from build123d import *

# Parameters (mm, degrees)
SKETCH1_R                       = 24.13
SKETCH1_R_2                     = 2.5
BOSS_EXTRUDE1_DEPTH             = 6.35
F_5_32_0_15625_DIAMETER_HOLE1_D = 3.96875


with BuildPart() as part:
    # Sketch1 → Boss-Extrude1 (new body)
    with BuildSketch(Plane(origin=(0, 0, 0), x_dir=(1, 0, 0), z_dir=(0, 1, 0))):
        Circle(SKETCH1_R)
        with Locations((19.2, 0)):
            Circle(SKETCH1_R_2, mode=Mode.SUBTRACT)
        with Locations((-9.6, 16.627687753)):
            Circle(SKETCH1_R_2, mode=Mode.SUBTRACT)
        with Locations((-9.6, -16.627687753)):
            Circle(SKETCH1_R_2, mode=Mode.SUBTRACT)
    extrude(amount=BOSS_EXTRUDE1_DEPTH)

    # 5/32 (0.15625) Diameter Hole1 (through all)
    with Locations(Plane(origin=(0, 6.35, 0), x_dir=(1, 0, 0), z_dir=(0, 1, 0))):
        with Locations((4.7625, 8.248891971), (-4.7625, 8.248891971), (-9.525, 0), (-4.7625, -8.248891971), (4.7625, -8.248891971), (9.525, 0)):
            Hole(F_5_32_0_15625_DIAMETER_HOLE1_D / 2)


solid = part.part
Build history of the part. All positions in model axes, mm. Give positions to 0.01 mm unless a question says otherwise; leave off trailing zeros. Order: outer loops, then holes, each group sorted by start corner. A loop starts at its lowest first (then second) coordinate and runs counter-clockwise, first axis right, second up. Notation, with made-up numbers: M 32.25,-14.75 L 44.25,-14.75 A19 ccw 44.25,4.25 Z; hole C 25.5,83 d3. An arc over 180 degrees is marked long. Use one line per item in the form item = value.
Q1. Pull direction X, two halves, no side cores. Call faces 1 (the cylindrical face through (5.021, 3.131, -10.216)), 2 (the cylindrical face through (23.016, 3.131, -7.248)), 3 (the flat face through (0, 6.35, 0)), 4 (the cylindrical face through (-7.543, 3.131, -0.087)): released by +X, released by -X, zero draft, split by the parting line, or undercut.
Conclusion:
face_1 = undercut
face_2 = split by the parting line
face_3 = zero draft
face_4 = undercut
Q2. Pin check, flat tips, straight feed: P1, Ø3.5, axis at x = 9.525, z = 0, coming from the -Y side; P2, Ø2, axis at y = 4, z = -3.5, coming from the -X side; P3, Ø1.5, axis at y = 4.5, z = 15.5, coming from the +X side. Stop position of each tip, or through.
Conclusion:
P1 = through
P2 = -24
P3 = 19.1
Q3. Slice it at B-B, the plane x = 18.5. Write the cut outline in (y, z), and give its area (3 significant figures).
Conclusion:
outline = M 0,-15.49 L 6.35,-15.49 L 6.35,-2.4 L 0,-2.4 Z; M 0,2.4 L 6.35,2.4 L 6.35,15.49 L 0,15.49 Z
area = 166 mm2
Q4. Slice it at A-A, the plane z = 0. Write the cut outline in (x, y), and give its area (3 significant figures).
Conclusion:
outline = M -24.13,0 L -11.51,0 L -11.51,6.35 L -24.13,6.35 Z; M -7.54,0 L 7.54,0 L 7.54,6.35 L -7.54,6.35 Z; M 11.51,0 L 16.7,0 L 16.7,6.35 L 11.51,6.35 Z; M 21.7,0 L 24.13,0 L 24.13,6.35 L 21.7,6.35 Z
area = 224 mm2
Q5. Slice it at C-C, the plane y = 2.75. State how many separate pieces and enclosed holes the cut face has, and give its area (3 significant figures).
Conclusion:
separate_pieces = 1
enclosed_holes = 9
area = 1,700 mm2
Q6. Wall check: probe 1 along Z at (x, y) = (10.5, 2.5); probe 2 along X at (y, z) = (4, -1.5); probe 3 along Z at (x, y) = (5, 2). Give the ranges that are in metal, low to high.
Conclusion:
probe_1 = -21.73 to -1.73, 1.73 to 21.73
probe_2 = -24.08 to -10.82, -8.23 to 8.23, 10.82 to 17.2, 21.2 to 24.08
probe_3 = -23.61 to -10.22, -6.28 to 6.28, 10.22 to 23.61
Q7. Slice it at D-D, the plane x = -5. Write the cut outline in (y, z).
Conclusion:
outline = M 0,-23.61 L 6.35,-23.61 L 6.35,-10.22 L 0,-10.22 Z; M 0,-6.28 L 6.35,-6.28 L 6.35,6.28 L 0,6.28 Z; M 0,10.22 L 6.35,10.22 L 6.35,23.61 L 0,23.61 Z
